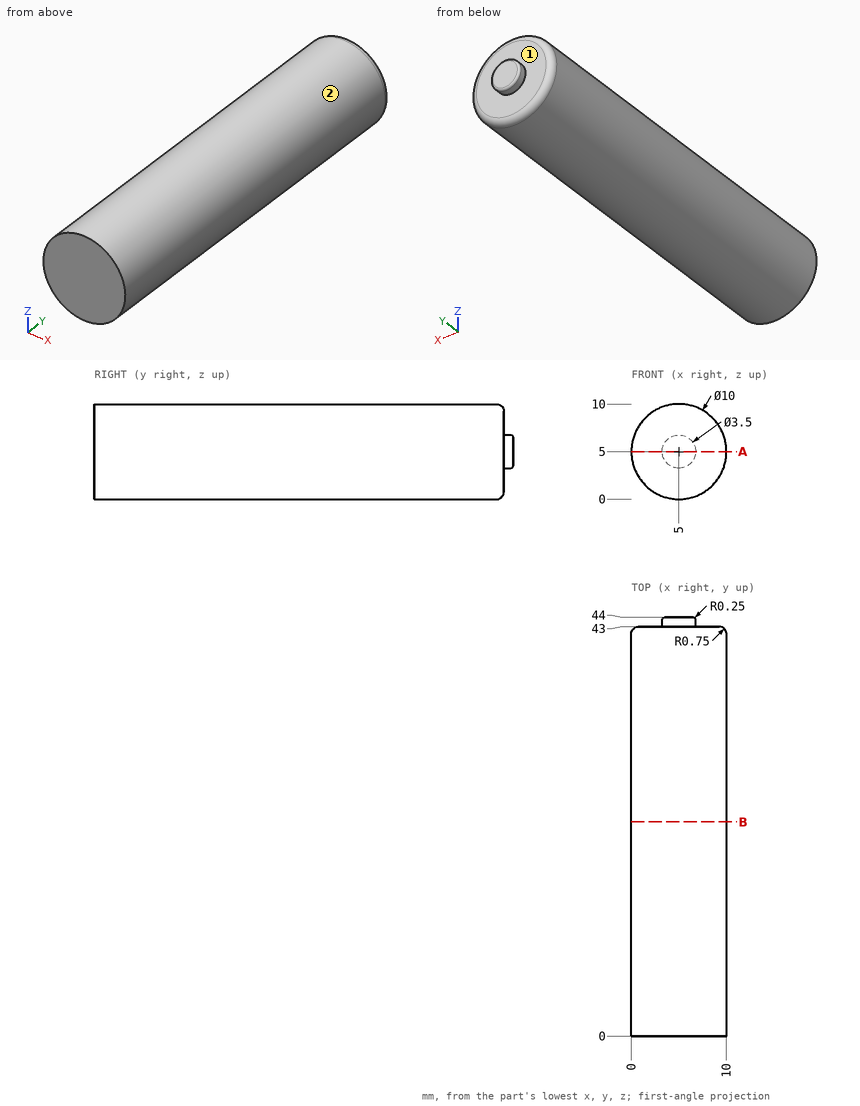
Can you work these out from the drawing? Everything is in mm from the part's minimum corner. A direction names the side the tool comes from. Round coordinates to 2 decimals unless told otherwise and drop trailing zeros. Write each loop counter-clockwise with the first axis right and the second up, starting at its lowest first coordinate (ties: lowest second). Pieces come first, ordered by that corner, then holes.
1. For the marked faces 1 and 2, which set-ups out of +Z, -Z, +X, -X, +Y, -Y let a thin tool reach every point of the face, with its end or its side?
2. Will these pins go through, and if not, where does the flat tip stop? pin 1 Ø2 at (x, y) = (2.5, 12.5) entering from -Z; pin 2 Ø2 at (x, y) = (1, 26.5) entering from +Z.
3. Suppose I cut it at A-A (z = 5). List the corners of the cut face in (x, y) for me, and give its area (3 significant figures).
4. Suppose I cut it at B-B (y = 22.5). List the corners of the cut face in (x, z) for me, and give its area (3 significant figures).
5. I need wall thicknesses on L1, parallel to Y at x = 8, z = 8; L2, parallel to Z at x = 4.75, y = 28. Which ranges of each line are inside material? Lowest first, please.
Answer sheet:
1. face 1: +Y
1. face 2: +Y, -Y
2. pin 1: stops at z = 0.23
2. pin 2: stops at z = 9
3. outline: (0, 0) - (10, 0) - (10, 42.25) arc R0.75 ccw to (9.25, 43) - (6.75, 43) - (6.75, 43.75) arc R0.25 ccw to (6.5, 44) - (3.5, 44) arc R0.25 ccw to (3.25, 43.75) - (3.25, 43) - (0.75, 43) arc R0.75 ccw to (0, 42.25) - close
3. area: 433 mm2
4. outline: circle Ø10 at (5, 5)
4. area: 78.5 mm2
5. L1: y = 0 to 43
5. L2: z = 0.01 to 9.99
